```python
from build123d import *

# Parameters (mm, degrees)
CHAMFER1_SIZE      = 0.6
CUT_EXTRUDE1_DEPTH = 3


with BuildPart() as part:
    # Sketch1 → Revolve1 (revolve)
    with BuildSketch(Plane.XY):
        Polygon((-6, 0), (-6, 4.4), (-5.4, 5), (0, 5), (0, 3), (12, 3), (12, 0), align=None)
    revolve(axis=Axis((12, 0, 0), (-1, 0, 0)))

    # Chamfer1
    chamfer1_edges = [part.edges().sort_by_distance(p)[0] for p in [
        (12, -3, 0),
    ]]
    chamfer(chamfer1_edges, length=CHAMFER1_SIZE)

    # Sketch2 → Cut-Revolve1 (revolve, cut)
    with BuildSketch(Plane.XY):
        Polygon((-6, 0), (-6, 2.5), (-3, 2.5), (-2.330127019, 0), align=None)
    revolve(axis=Axis((-2.330127019, 0, 0), (-1, 0, 0)), mode=Mode.SUBTRACT)

    # Sketch3 → Cut-Extrude1 (cut)
    with BuildSketch(Plane(origin=(-6, 0, 0), x_dir=(0, 0, -1), z_dir=(1, 0, 0))):
        Polygon((-2.5, 1.443375673), (-2.5, -1.443375673), (0, -2.886751346), (2.5, -1.443375673), (2.5, 1.443375673), (0, 2.886751346), align=None)
    extrude(amount=CUT_EXTRUDE1_DEPTH, mode=Mode.SUBTRACT)


solid = part.part
```
Can you work these out from the model? Positions are in its coordinate system, mm. A direction names the side the tool comes from. Coordinates: 2 decimals unless noted, no trailing zeros. Write each loop counter-clockwise with the first axis right and the second up, starting at its lowest first coordinate (ties: lowest second). Pieces come first, ordered by that corner, then holes. Notation, with made-up numbers: M -38.5,47 L -8.5,47 A13 cw -8.5,66 Z; hole C -6.75,-0.5 d7. An arc over 180 degrees is marked long. Answer as CSV lines item,"result".
Item 1: I'm going to push flat-ended pins straight in: P1, Ø1, axis at y = 3, z = -3, coming from the +X side; P2, Ø1.4, axis at x = -4.5, y = -0.5, coming from the -Z side; P3, Ø1.5, axis at x = 8, y = -2.5, coming from the +Z side; P4, Ø5, axis at x = 9, y = -2.5, coming from the -Z side. Where does each tip first touch, or does it pass through?
Geometry results:
P1,"stops at x = 0"
P2,"stops at z = -5"
P3,"stops at z = 2.44"
P4,"stops at z = -3"
Item 2: On a 3-axis mill with a long thin cutter (end or side, diameter ignored), from which of +Z, -Z, +X, -X, +Y, -Y can I reach the whole of each face in a straight line? I mean faces 5 (the flat face through (0, 3.3, -0.1)), 6 (the cylindrical face through (-2.66, -1.08, 4.88)), 7 (the flat face through (-4.521, 2.155, -1.267)). Say none if no direction works.
Geometry results:
face 5,"+X"
face 6,"+X, -X"
face 7,"-X"
Item 3: Imagine slicing it at A-A on x = 4. List the corners of the cut face in (y, z) for me.
Geometry results:
outline,"C 0,0 d6"
Item 4: Please list where these lines run through material, in increasing order: line 1 along X through (y, z) = (-2.75, -1.75); line 2 along Y through (x, z) = (8.5, 1.5); line 3 along Y through (x, z) = (11, -0.5).
Geometry results:
line 1,"x = -6 to 0"
line 2,"y = -2.6 to 2.6"
line 3,"y = -2.96 to 2.96"
Item 5: We'd pull the mould along Z, two halves only. Please class faces 1 (the cylindrical face through (6, -3, 0)), 2 (the flat face through (-4.521, -2.175, -1.233)), 3 (the flat face through (-6, -2, 2)), 4 (the flat face through (-4.521, -2.155, 1.267)): +Z half, -Z half, draft (parallel to the pull), parting line (faces both ways), or undercut.
Geometry results:
face 1,"parting line"
face 2,"undercut"
face 3,"draft"
face 4,"undercut"
